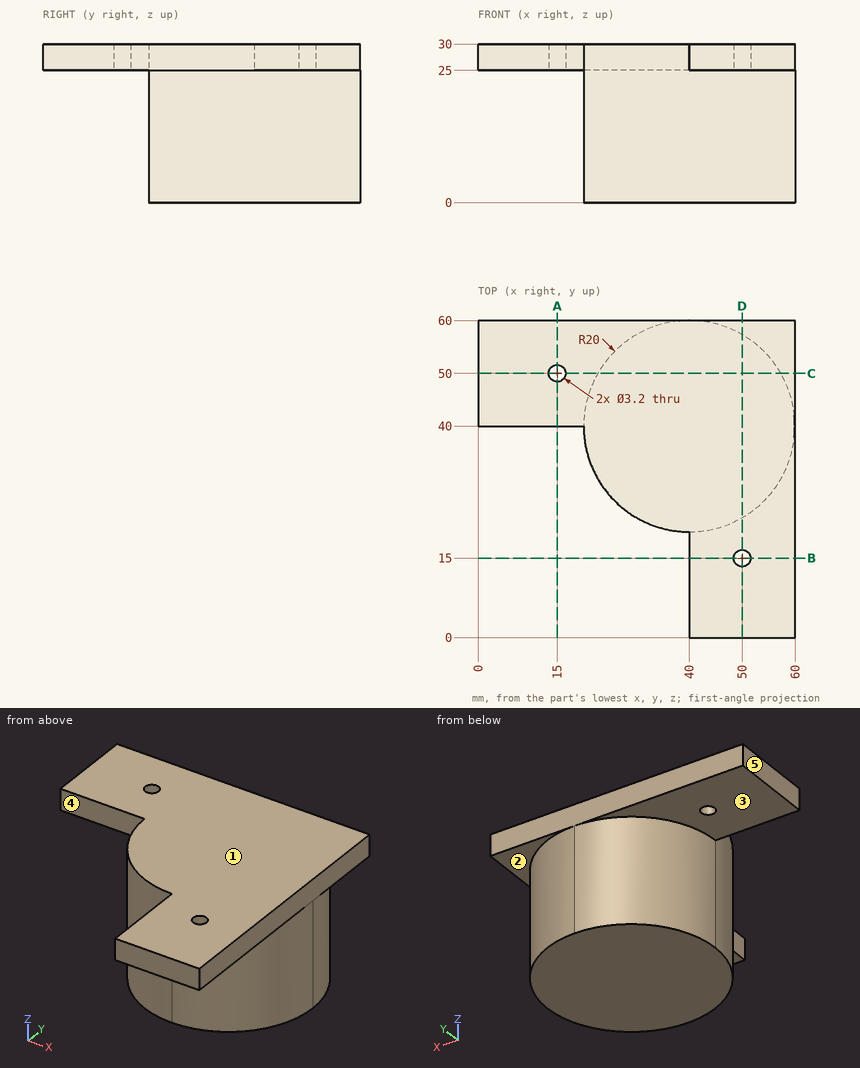
Answer from the drawing. Dimensions are ordinates in mm from the lowest x, y and z of the part. A direction names the side the tool comes from. Give positions to 0.01 mm unless a question says otherwise; leave off trailing zeros. Loops run counter-clockwise (first coordinate to the right, second up) from the corner with the lowest first, then second, coordinate; pieces in that order, holes last. Notation, with made-up numbers: (80, -4.75) -> (94, -4.75) arc R12 cw to (94, 8.25) -> close; hole circle Ø2 at (-28.5, -12). An arc over 180 degrees is marked (long way). One line per question, with ' | ' between items. Start each with the question number.
1) Section C-C, the plane y = 50 is taken. Determine the outline of the cut face in (x, z).
2) For the marked faces 1, 2, 3, 4 and 5, determine the directions among +Z, -Z, +X, -X, +Y, -Y from which every point of the face is accessible in a straight line to the end or side of a thin tool.
3) Each of these flat-tipped pins is pushed along its axis until it touches: pin 1 (3 mm diameter, centred on x = 35, z = 24.5, fed in from -Y); pin 2 (2 mm diameter, centred on y = 49.5, z = 7.5, fed in from +X); pin 3 (1.5 mm diameter, centred on y = 11, z = 28.5, fed in from -X). Where does it stop, or does it pass through?
4) Straight lines are drawn through the part: L1, parallel to Y at x = 50, z = 28.65; L2, parallel to Y at x = 15, z = 27.8; L3, parallel to Z at x = 55.5, y = 15. For each, find the intervals that lie inside material, in ascending order.
5) Section A-A, the plane x = 15 is taken. Determine the outline of the cut face in (y, z), then the cut area to 3 significant figures.
Resolved:
1) outline: (0, 25) -> (13.4, 25) -> (13.4, 30) -> (0, 30) -> close; (16.6, 25) -> (22.68, 25) -> (22.68, 0) -> (57.32, 0) -> (57.32, 25) -> (60, 25) -> (60, 30) -> (16.6, 30) -> close
2) face 1: +Z, +X, -X, +Y, -Y | face 2: -Z, +X, +Y | face 3: -Z, -X, +Y | face 4: +Z, -Z, -X, -Y | face 5: +Z, -Z, -X, +Y, -Y
3) pin 1: y = 20.31 | pin 2: x = 58.1 | pin 3: x = 40
4) L1: 0 to 13.4, 16.6 to 60 | L2: 40 to 48.4, 51.6 to 60 | L3: 25 to 30
5) outline: (40, 25) -> (48.4, 25) -> (48.4, 30) -> (40, 30) -> close; (51.6, 25) -> (60, 25) -> (60, 30) -> (51.6, 30) -> close | area: 84.0 mm2
